Autodesk Inventor part; units mm, degrees
ref_plane "YZ Plane" through (0, 0, 0) normal (1, 0, 0) x (0, 1, 0)
ref_plane "XZ Plane" through (0, 0, 0) normal (0, 1, 0) x (-1, 0, 0)
ref_plane "XY Plane" through (0, 0, 0) normal (0, 0, 1) x (1, 0, 0)
sketch "Sketch1" plane through (0, 0, 0) normal (0, 1, 0) x (-1, 0, 0)
  line L0 (5.1091, 9.9192) -> (-42.0909, 9.9192)
  line L1 (-42.0909, 9.9192) -> (-42.0909, -13.5608)
  line L2 (-42.0909, -13.5608) -> (5.1091, -13.5608)
  line L3 (5.1091, -13.5608) -> (5.1091, 9.9192)
  point P0 (0, 0)
  dimension "d0" = 23.48
  dimension "d1" = 47.2
extrude "Extrusion1" add sketch "Sketch1" along normal blind 5.31
sketch "Sketch2" plane through (0, 5.31, 0) normal (0, 1, 0) x (1, 0, 0)
  circle A0 centre (-0.1791, 1.8208) radius 0.93
  circle A1 centre (5.4509, -5.2092) radius 0.93
  line L0 (-5.1091, -9.9192) -> (42.0909, -9.9192)
  line L1 (42.0909, 13.5608) -> (-5.1091, 13.5608)
  circle A2 centre (5.4509, 8.8508) radius 0.93
  line L2 (-5.1091, 13.5608) -> (-5.1091, -9.9192)
  line L3 (42.0909, -9.9192) -> (42.0909, 13.5608)
  circle A3 centre (37.1609, 1.8208) radius 0.93
  point P0 (0, 0)
  dimension "d4" = 1.86
  dimension "d7" = 1.86
  dimension "d10" = 3.78
  dimension "d12" = 0
  dimension "d14" = 1.86
  dimension "d15" = 14.06
  dimension "d16" = 3.78
  dimension "d17" = 4
  dimension "d19" = 0
  dimension "d20" = 1.86
  dimension "d23" = 37.34
  dimension "d24" = 4
  dimension "d27" = 5.63
  dimension "d29" = 11.74
  dimension "d30" = 11.74
extrude "Extrusion2" cut sketch "Sketch2" against normal through all contours A0 | A1 | A2 | A3
sketch "Sketch3" plane through (0, 5.31, 0) normal (0, 1, 0) x (1, 0, 0)
  line L0 (1.7509, -3.2792) -> (35.2309, -3.2792)
  line L1 (35.2309, -3.2792) -> (35.2309, 6.9208)
  line L2 (35.2309, 6.9208) -> (1.7509, 6.9208)
  line L3 (1.7509, 6.9208) -> (1.7509, -3.2792)
  circle A0 centre (-0.1791, 1.8208) radius 0.93
  circle A1 centre (5.4509, 8.8508) radius 0.93
  circle A2 centre (5.4509, -5.2092) radius 0.93
  circle A3 centre (37.1609, 1.8208) radius 0.93
  point P0 (0, 0)
  dimension "d33" = 1
  dimension "d34" = 1
  dimension "d35" = 1
  dimension "d36" = 1
extrude "Extrusion3" cut sketch "Sketch3" against normal through all contours L3 L2 L1 L0
properties part number "490HV_SampleConnector"
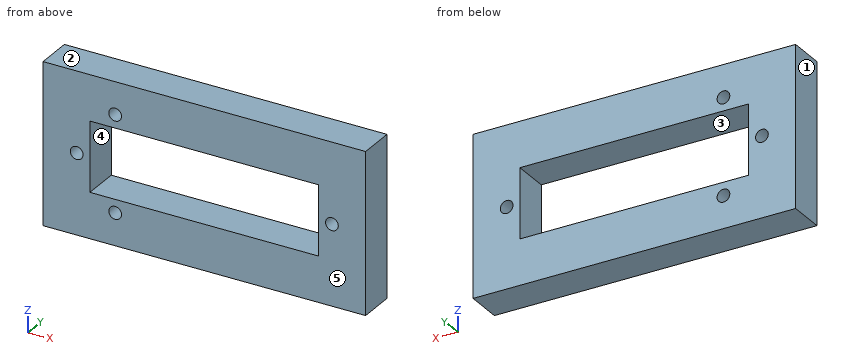
Here's how the part is built. I have some questions about the finished solid (model axes, mm). Face numbers are marked on the shaded views. A direction names the side the tool comes from. Round coordinates to 2 decimals unless told otherwise and drop trailing zeros. Write each loop counter-clockwise with the first axis right and the second up, starting at its lowest first coordinate (ties: lowest second). Pieces come first, ordered by that corner, then holes.
Q1. If we section it at A-A on z = -4.25: Write out the boundary of the cut face in (x, y).
Q2. Please list where these lines run through material, in increasing order: probe 1 along Z at (x, y) = (5.5, 3.8); probe 2 along Z at (x, y) = (25.5, 1.65); probe 3 along X at (y, z) = (2.5, 2).
Q3. If we mould it in two halves opening along X, with no side actions, what happens to the marked faces 1, 2 and 3? For each: +X half, -X half, draft (parallel to the pull), parting line (faces both ways), or undercut.
Q4. If we section it at C-C on y = 0.5: Write out the boundary of the cut face in (x, z), plus the area to 3 significant figures.
Q5. If we section it at B-B on x = 15.5: Write out the boundary of the cut face in (y, z), plus the area to 3 significant figures.
Q6. Which directions (+Z, -Z, +X, -X, +Y, -Y) give clear straight access to the entire face, cutting with the end or side of a thin tool? Please do the marked faces 4 and 5.
Answer below:
1. outline: (-5.11, 0) - (1.75, 0) - (1.75, 5.31) - (-5.11, 5.31) - close; (35.23, 0) - (42.09, 0) - (42.09, 5.31) - (35.23, 5.31) - close
2. probe 1: z = -13.56 to -9.78, -7.92 to -6.92, 3.28 to 4.28, 6.14 to 9.92
2. probe 2: z = -13.56 to -6.92, 3.28 to 9.92
2. probe 3: x = -5.11 to 1.75, 35.23 to 42.09
3. face 1: -X half
3. face 2: draft
3. face 3: undercut
4. outline: (-5.11, -13.56) - (42.09, -13.56) - (42.09, 9.92) - (-5.11, 9.92) - close; hole circle Ø1.86 at (-0.18, -1.82); hole (1.75, -6.92) - (35.23, -6.92) - (35.23, 3.28) - (1.75, 3.28) - close; hole circle Ø1.86 at (5.45, -8.85); hole circle Ø1.86 at (5.45, 5.21); hole circle Ø1.86 at (37.16, -1.82)
4. area: 756 mm2
5. outline: (0, -13.56) - (5.31, -13.56) - (5.31, -6.92) - (0, -6.92) - close; (0, 3.28) - (5.31, 3.28) - (5.31, 9.92) - (0, 9.92) - close
5. area: 70.5 mm2
6. face 4: +Y, -Y
6. face 5: +Z, -Z, +X, -X, -Y
